Build history of the part. All positions in model axes, mm. A direction names the side the tool comes from. Round coordinates to 2 decimals unless told otherwise and drop trailing zeros. Write each loop counter-clockwise with the first axis right and the second up, starting at its lowest first coordinate (ties: lowest second). Pieces come first, ordered by that corner, then holes.
1) Saw through at D-D (x = 14.5). Write the cut outline in (y, z).
2) Flat gauge pins, fed straight in: pin 1 (16.5 mm diameter, centred on x = 50.5, y = -61.5, fed in from +Z); pin 2 (10 mm diameter, centred on x = 105.5, z = 62, fed in from +Y); pin 3 (22.5 mm diameter, centred on y = -45.5, z = 55.5, fed in from -X); pin 4 (4.5 mm diameter, centred on x = 129, y = -42, fed in from +Z). Where does each tip first touch, or does it go through?
3) Saw through at A-A (x = 93.98). Write the cut outline in (y, z).
4) Wall check: probe 1 along Y at (x, z) = (9.5, 26); probe 2 along Z at (x, y) = (93, -42); probe 3 along X at (y, z) = (-19, 20). Give the ranges that are in metal, low to high.
5) Pull direction X, two halves, no side cores. Call faces 1 (the flat face through (129, -38, 43.18)), 2 (the flat face through (138, -38, 71.12)), 3 (the cylindrical face through (2.897, -73.145, 17.531)): +X half, -X half, draft (parallel to the pull), parting line (faces both ways), or undercut.
6) Which spindle directions (+Z, -Z, +X, -X, +Y, -Y) get a long thin tool onto all of the face, cutting with end or side? Do faces 4 (the flat face through (16, -43.18, 29)), 5 (the flat face through (39, -59, 35.56)), 6 (the flat face through (137.16, -38, 57)). Say none if no direction does.
7) Saw through at C-C (x = 129.54). Write the cut outline in (y, z).
8) Saw through at B-B (y = -37.5). Write the cut outline in (x, z).
from build123d import *

# Parameters (mm, degrees)
F1_DEPTH  = 76.2
F2_R      = 10.16
F3_R      = 10.16
F4_DEPTH  = 76.201
F6_DEPTH  = 27.94
F7_W      = 76.2
F7_H      = 10.16
F8_DEPTH  = 10.16
F9_R      = 7.62
F9_R_2    = 3.175
F10_DEPTH = 10.16
F11_DEPTH = 4.064


with BuildPart() as f1:
    # F0 (on Front) → F1 (new body)
    with BuildSketch(Plane.XZ):
        Polygon((0, 35.56), (0, 0), (111.76, 0), (147.32, 35.56), (147.32, 71.12), (111.76, 71.12), (76.2, 35.56), align=None)
    extrude(amount=F1_DEPTH)

    # F2
    f2_edges = [f1.edges().sort_by_distance(p)[0] for p in [
        (0, -76.2, 17.78),
        (0, 0, 17.78),
    ]]
    fillet(f2_edges, radius=F2_R)

    # F3 (on face) → F4 (cut, through all)
    with BuildSketch(Plane.XZ):
        with Locations((93.98, 20.32)):
            Circle(F3_R)
    extrude(amount=F4_DEPTH, mode=Mode.SUBTRACT)

    # F5 (on face) → F6 (cut)
    with BuildSketch(Plane.XY.offset(71.12)):
        with BuildLine():
            ThreePointArc((137.16, -15.24), (129.54, -7.62), (121.92, -15.24))
            Line((121.92, -15.24), (121.92, -60.96))
            ThreePointArc((121.92, -60.96), (129.54, -68.58), (137.16, -60.96))
            Line((137.16, -60.96), (137.16, -15.24))
        make_face()
    extrude(amount=-F6_DEPTH, mode=Mode.SUBTRACT)

    # F7 (on face) → F8 (cut)
    with BuildSketch(Plane.XY.offset(35.56)):
        with Locations((38.1, -38.1)):
            Rectangle(F7_W, F7_H)
    extrude(amount=-F8_DEPTH, mode=Mode.SUBTRACT)

    # F9 (on face) → F10 (cut)
    with BuildSketch(Plane.XY.offset(35.56)):
        with Locations((38.1, -38.1)):
            Circle(F9_R)
        with Locations((38.1, -38.1)):
            Circle(F9_R_2, mode=Mode.SUBTRACT)
    extrude(amount=-F10_DEPTH, mode=Mode.SUBTRACT)

    # F9 (on face) + F10_face (on face) → F11 (cut)
    with BuildSketch(Plane.XY.offset(35.56)):
        with Locations((38.1, -38.1)):
            Circle(F9_R)
        with Locations((38.1, -38.1)):
            Circle(F9_R_2, mode=Mode.SUBTRACT)
    with BuildSketch(Plane(origin=(38.1, -38.1, 25.4), x_dir=(1, 0, 0), z_dir=(0, 0, 1))):
        with BuildLine():
            Line((-38.1, -5.08), (-5.679613, -5.08))
            ThreePointArc((-5.679613, -5.08), (0, -7.62), (5.679613, -5.08))
            Line((5.679613, -5.08), (38.1, -5.08))
            Line((38.1, -5.08), (38.1, 5.08))
            Line((38.1, 5.08), (5.679613, 5.08))
            ThreePointArc((5.679613, 5.08), (0, 7.62), (-5.679613, 5.08))
            Line((-5.679613, 5.08), (-38.1, 5.08))
            Line((-38.1, 5.08), (-38.1, -5.08))
        make_face()
    extrude(amount=-F11_DEPTH, mode=Mode.SUBTRACT)


solid = f1.part
Evaluation:
1. outline: (-76.2, 0) - (0, 0) - (0, 35.56) - (-33.02, 35.56) - (-33.02, 21.34) - (-43.18, 21.34) - (-43.18, 35.56) - (-76.2, 35.56) - close
2. pin 1: stops at z = 35.56
2. pin 2: stops at y = 0
2. pin 3: stops at x = 84.89
2. pin 4: stops at z = 43.18
3. outline: (-76.2, 0) - (0, 0) - (0, 10.16) - (-76.2, 10.16) - close; (-76.2, 30.48) - (0, 30.48) - (0, 53.34) - (-76.2, 53.34) - close
4. probe 1: y = -76.18 to -43.18, -33.02 to -0.02
4. probe 2: z = 0 to 10.21, 30.43 to 52.36
4. probe 3: x = 0 to 83.83, 104.13 to 131.76
5. face 1: undercut
5. face 2: draft
5. face 3: -X half
6. face 4: +Z, -X
6. face 5: +Z, -X, +Y, -Y
6. face 6: +Z
7. outline: (-76.2, 17.78) - (0, 17.78) - (0, 71.12) - (-7.62, 71.12) - (-7.62, 43.18) - (-68.58, 43.18) - (-68.58, 71.12) - (-76.2, 71.12) - close
8. outline: (0, 0) - (111.76, 0) - (147.32, 35.56) - (147.32, 71.12) - (137.16, 71.12) - (137.16, 43.18) - (121.92, 43.18) - (121.92, 71.12) - (111.76, 71.12) - (76.2, 35.56) - (76.2, 21.34) - (0, 21.34) - close; hole circle Ø20.32 at (93.98, 20.32)
